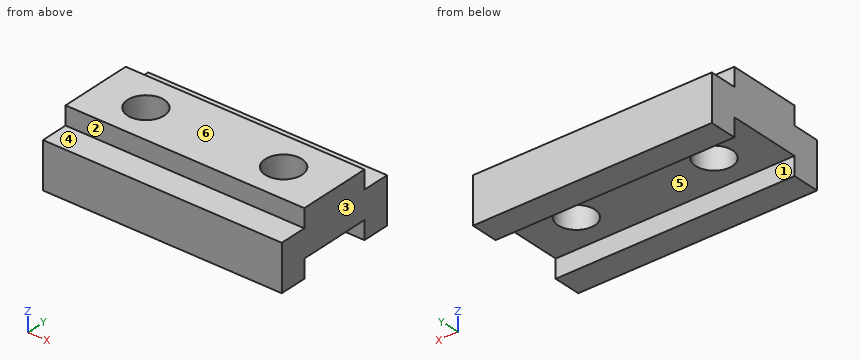
from build123d import *

# Parameters (mm, degrees)
F1_DEPTH = 165.1
F4_DEPTH = 44.451


with BuildPart() as f1:
    # F0 (on Right) → F1 (new body)
    with BuildSketch(Plane.YZ):
        Polygon((-25.4, 0), (0, 0), (25.4, 0), (25.4, -12.7), (44.45, -12.7), (44.45, 19.05), (25.4, 19.05), (25.4, 31.75), (-25.4, 31.75), (-25.4, 19.05), (-44.45, 19.05), (-44.45, -12.7), (-25.4, -12.7), align=None)
    extrude(amount=F1_DEPTH)

    # F3 (on face) → F4 (cut, through all)
    with BuildSketch(Plane.XY.offset(31.75)):
        with BuildLine():
            Line((34.925, 0), (47.496461463, 0))
            ThreePointArc((47.496461463, 0), (34.796461463, 12.7), (22.096461463, 0))
            Line((22.096461463, 0), (34.925, 0))
        make_face()
        with BuildLine():
            ThreePointArc((22.096461463, 0), (34.796461463, -12.7), (47.496461463, 0))
            Line((47.496461463, 0), (34.925, 0))
            Line((34.925, 0), (22.096461463, 0))
        make_face()
        with BuildLine():
            ThreePointArc((142.6928426743, 0), (129.9928426743, 12.7), (117.2928426743, 0))
            ThreePointArc((117.2928426743, 0), (129.9928426743, -12.7), (142.6928426743, 0))
        make_face()
    extrude(amount=-F4_DEPTH, mode=Mode.SUBTRACT)


solid = f1.part
For this review, take the finished solid that the model builds, in its own axes (mm). Face numbers are marked on the shaded views. A direction names the side the tool comes from. Give positions to 0.01 mm unless a question says otherwise; leave off trailing zeros. Loops run counter-clockwise (first coordinate to the right, second up) from the corner with the lowest first, then second, coordinate; pieces in that order, holes last. Notation, with made-up numbers: M 35,-9.5 L 39,-9.5 A23 ccw 39,21.5 Z; hole C 89.25,55.5 d6. An arc over 180 degrees is marked long. Answer as a JSON object with one key per item and string values. Group by question number.
Q1. Mouldability with a two-part tool opening along Y and no side actions: class the marked faces 1, 2 and 3 as +Y half, -Y half, draft (parallel to the pull), parting line (faces both ways), or undercut.
Q2. Tool access review of the marked faces 4, 5 and 6: name each direction out of +Z, -Z, +X, -X, +Y, -Y from which nothing blocks a thin tool from reaching the whole face with its end or side.
Q3. For probe 1 along Y at (x, z) = (34, -0.5); probe 2 along Y at (x, z) = (34, 24.5) (3 decimals); probe 3 along X at (y, z) = (1, 4.5), list the stretches that pass through material, from the lowest coordinate up. Write a range as [from, to].
Q4. Add section A-A on z = -7.5. Give the boundary of the cut face in (x, y).
Q5. Add section D-D on z = 6. Give the boundary of the cut face in (x, y), and give its area (3 significant figures).
Q6. Add section C-C on x = 19.5. Give the boundary of the cut face in (y, z).
Q7. Insertion check: P1, Ø14, axis at x = 53, z = 23, coming from the +Y side; P2, Ø10, axis at x = 72.5, z = 25, coming from the -Y side; P3, Ø15, axis at x = 52.5, y = 33.5, coming from the +Z side; P4, Ø3, axis at x = 58.5, y = 12, coming from the -Z side. Each pin has a flat end and moves straight along its axis. Give the tip position at first contact, or say it passes through.
Q8. Add section B-B on y = -4. Give the boundary of the cut face in (x, z).
Checked values:
{
 "1": {"face 1": "undercut", "face 2": "-Y half", "face 3": "draft"},
 "2": {"face 4": "+Z, +X, -X, -Y", "face 5": "-Z, +X, -X", "face 6": "+Z, +X, -X, +Y, -Y"},
 "3": {"probe 1": "[-44.45, -25.4], [25.4, 44.45]", "probe 2": "[-25.4, -12.675], [12.675, 25.4]", "probe 3": "[0, 22.14], [47.46, 117.33], [142.65, 165.1]"},
 "4": {"outline": "M 0,-44.45 L 165.1,-44.45 L 165.1,-25.4 L 0,-25.4 Z; M 0,25.4 L 165.1,25.4 L 165.1,44.45 L 0,44.45 Z"},
 "5": {"outline": "M 0,-44.45 L 165.1,-44.45 L 165.1,44.45 L 0,44.45 Z; hole C 34.8,0 d25.4; hole C 129.99,0 d25.4", "area": "13,700 mm²"},
 "6": {"outline": "M -44.45,-12.7 L -25.4,-12.7 L -25.4,0 L 25.4,0 L 25.4,-12.7 L 44.45,-12.7 L 44.45,19.05 L 25.4,19.05 L 25.4,31.75 L -25.4,31.75 L -25.4,19.05 L -44.45,19.05 Z"},
 "7": {"P1": "y = 44.45", "P2": "y = -25.4", "P3": "z = 19.05", "P4": "z = 0"},
 "8": {"outline": "M 0,0 L 22.74,0 L 22.74,31.75 L 0,31.75 Z; M 46.85,0 L 117.94,0 L 117.94,31.75 L 46.85,31.75 Z; M 142.05,0 L 165.1,0 L 165.1,31.75 L 142.05,31.75 Z"}
}
